Design review of the part built by this model. Coordinates are the model's own, in mm. A direction names the side the tool comes from. Give positions to 0.01 mm unless a question says otherwise; leave off trailing zeros. Order: outer loops, then holes, each group sorted by start corner. A loop starts at its lowest first (then second) coordinate and runs counter-clockwise, first axis right, second up. Notation, with made-up numbers: M -5.75,-19 L 23.25,-19 A14 ccw 23.25,-3 Z; hole C 74,47.25 d1. An arc over 180 degrees is marked long. Answer as a JSON object with one key per item and string values.
Autodesk Inventor part; units mm, degrees
ref_plane "YZ Plane" through (0, 0, 0) normal (1, 0, 0) x (0, 1, 0)
ref_plane "XZ Plane" through (0, 0, 0) normal (0, 1, 0) x (-1, 0, 0)
ref_plane "XY Plane" through (0, 0, 0) normal (0, 0, 1) x (1, 0, 0)
sketch "Sketch1" plane through (0, 0, 0) normal (0, 1, 0) x (-1, 0, 0)
  line L0 (4, 35) -> (-4, 35)
  line L1 (-4, 35) -> (-4, -35)
  line L2 (-4, -35) -> (4, -35)
  line L3 (4, -35) -> (4, 35)
  line L4 (4, 35) -> (-4, -35) construction
  line L5 (-4, 35) -> (4, -35) construction
  circle A0 centre (15, 0) radius 15
  arc A1 (4, 22.2261) -> (12.6667, 14.8174) centre (11.5, 22.2261) ccw
  arc A2 (12.6667, -14.8174) -> (4, -22.2261) centre (11.5, -22.2261) ccw
  point P0 (0, 0)
  dimension "d0" = 8
  dimension "d1" = 70
  dimension "d2" = 30
  dimension "d3" = 15
  dimension "d6" = 15
  dimension "d7" = 7.5
  dimension "d9" = 0
  dimension "d10" = 15
extrude "Extrusion1" add sketch "Sketch1" along normal blind 10
sketch "Sketch2" plane through (0, 10, 0) normal (0, 1, 0) x (1, 0, 0)
  circle A0 centre (-15, 0) radius 11.125
  arc A1 (-12.6667, 14.8174) -> (-12.6667, -14.8174) centre (-15, 0) ccw
  point P0 (0, 0)
  dimension "d13" = 22.25
extrude "Extrusion2" cut sketch "Sketch2" against normal blind 7
sketch "Sketch3" plane through (-15, 3, 0) normal (0, 1, 0) x (1, 0, 0)
  circle A0 centre (0, 0) radius 10.5
  point P0 (15, 0)
  dimension "d16" = 21
extrude "Extrusion3" cut sketch "Sketch3" against normal blind 7
sketch "Sketch4" plane through (-4, 0, 22.2261) normal (-1, 0, 0) x (0, 0, 1)
  circle A0 centre (6.7739, 5) radius 3
  line L0 (0, 0) -> (12.7739, 0)
  line L1 (12.7739, 0) -> (12.7739, 10)
  circle A1 centre (-51.2261, 5) radius 3
  line L2 (-57.2261, 10) -> (-44.4522, 10)
  line L3 (-57.2261, 0) -> (-57.2261, 10)
  point P0 (-22.2261, 0)
  point P1 (6.3869, 0)
  dimension "d19" = 6
  dimension "d20" = 5
  dimension "d21" = 6
  dimension "d22" = 6
  dimension "d23" = 5
  dimension "d24" = 6
extrude "Extrusion4" cut sketch "Sketch4" against normal blind 7
properties part number "Bearing Holder"
(1) Draft analysis for pull direction Z (two halves, no side actions). For faces 6 (the cylindrical face through (-6.696, 4.93, 16.467)), 7 (the flat face through (3, 5, 29)), 8 (the cylindrical face through (-30, 5, 0)), 9 (the flat face through (-4, 4.9, 25.7)), state which applies: +Z half, -Z half, draft (parallel to the pull), parting line (faces both ways), or undercut.
Checked values:
{"face 6": "+Z half", "face 7": "undercut", "face 8": "parting line", "face 9": "draft"}
(2) To check wall thickness, follow L1, parallel to Z at x = -15.5, y = 7.5; L2, parallel to X at y = 2.35, z = 0; L3, parallel to Y at x = 0, z = -29. State the ranges of each line that lie inside material, in increasing order. Write a range as from..to.
Checked values:
{"L1": "z = -14.99..-11.11, 11.11..14.99", "L2": "x = -30..-25.5, -4.5..4", "L3": "y = 0..2, 8..10"}
(3) Tool access review of faces 1 (the flat face through (-11, 3, 10)), 2 (the flat face through (-4, 4, -26)), 3 (the flat face through (4, 5, 0)), 4 (the flat face through (3, 5, -29)), 5 (the cylindrical face through (-6.558, 4.93, -16.585)): name each direction out of +Z, -Z, +X, -X, +Y, -Y from which nothing blocks a thin tool from reaching the whole face with its end or side.
Checked values:
{"face 1": "+Y", "face 2": "-Z, -X, +Y, -Y", "face 3": "+Z, -Z, +X, +Y, -Y", "face 4": "-X", "face 5": "-Z, +Y, -Y"}
(4) We need section A-A (z = 0). Write out the cut boundary in (x, y) (3 decimals).
Checked values:
{"outline": "M -30,0 L -25.5,0 L -25.5,3 L -26.125,3 L -26.125,10 L -30,10 Z; M -4.5,0 L 4,0 L 4,10 L -3.875,10 L -3.875,3 L -4.5,3 Z"}
(5) We need section B-B (x = -15). Write out the cut boundary in (y, z) (3 decimals).
Checked values:
{"outline": "M 0,-15 L 10,-15 L 10,-11.125 L 3,-11.125 L 3,-10.5 L 0,-10.5 Z; M 0,10.5 L 3,10.5 L 3,11.125 L 10,11.125 L 10,15 L 0,15 Z"}
(6) Insertion check: pin 1 (5 mm diameter, centred on y = 7.5, z = -25.5, fed in from -X); pin 2 (1.8 mm diameter, centred on y = 5, z = -28.5, fed in from -X); pin 3 (3 mm diameter, centred on y = 3, z = -5.5, fed in from -X); pin 4 (18 mm diameter, centred on x = -15, z = 0, fed in from -Y). Each pin has a flat end and moves straight along its axis. Give the tip position at first contact, or say it passes through.
Checked values:
{"pin 1": "stops at x = -4", "pin 2": "stops at x = 3", "pin 3": "stops at x = -29.46", "pin 4": "passes through"}
(7) We need section C-C (z = 29). Write out the cut boundary in (x, y).
Checked values:
{"outline": "M -4,0 L 4,0 L 4,10 L -4,10 L -4,8 L 3,8 L 3,2 L -4,2 Z"}
